Source: CAD feature listing. Evaluate the final solid. Frame: model axes, mm. A direction names the side the tool comes from. Coordinates: 2 decimals unless noted, no trailing zeros. Loops run counter-clockwise (first coordinate to the right, second up) from the corner with the lowest first, then second, coordinate; pieces in that order, holes last.
from build123d import *

# Parameters (mm, degrees)
SKETCH1_W               = 3.175
SKETCH1_H               = 76.2
BOSS_EXTRUDE1_DEPTH     = 12.7
BOSS_EXTRUDE1_2_DEPTH   = 12.7
SKETCH1_3_W             = 12.7
SKETCH1_3_H             = 76.2
SKETCH1_3_W_2           = 3.175
BOSS_EXTRUDE2_DEPTH     = 3.175
FILLET1_R               = 6.35
SKETCH2_W               = 3.175
SKETCH2_H               = 76.2
BOSS_EXTRUDE3_DEPTH     = 9.525
CUT_EXTRUDE1_DEPTH      = 47.878313216
CUT_EXTRUDE1_DEPTH_BACK = 47.878313216
SKETCH3_R               = 2.032
SKETCH4_R               = 1.905
CUT_EXTRUDE2_DEPTH      = 3.175


with BuildPart() as part:
    # Sketch1 → Boss-Extrude1 (new body)
    with BuildSketch(Plane.XY):
        with Locations((-7.9375, 0)):
            Rectangle(SKETCH1_W, SKETCH1_H)
    extrude(amount=BOSS_EXTRUDE1_DEPTH)



with BuildPart() as body_2:
    # Sketch1 → Boss-Extrude1 2 (new body)
    with BuildSketch(Plane.XY):
        with Locations((7.9375, 0)):
            Rectangle(SKETCH1_W, SKETCH1_H)
    extrude(amount=BOSS_EXTRUDE1_2_DEPTH)


with BuildPart() as part_1:
    add(part.part)

    add(body_2.part)  # Boss-Extrude2 merges body 2
    # Sketch1<3> → Boss-Extrude2 (add)
    with BuildSketch(Plane.XY):
        Rectangle(SKETCH1_3_W, SKETCH1_3_H)
        with Locations((7.9375, 0)):
            Rectangle(SKETCH1_3_W_2, SKETCH1_3_H)
        with Locations((-7.9375, 0)):
            Rectangle(SKETCH1_3_W_2, SKETCH1_3_H)
    extrude(amount=-BOSS_EXTRUDE2_DEPTH)

    # Fillet1
    fillet1_edges = [part_1.edges().sort_by_distance(p)[0] for p in [
        (6.35, 0, 0),
        (-6.35, 0, 0),
    ]]
    fillet(fillet1_edges, radius=FILLET1_R - 0.0001)  # a hair under: the kernel refuses the full size

    # Sketch2 → Boss-Extrude3 (add)
    with BuildSketch(Plane.XY.offset(12.7)):
        with Locations((-7.9375, 0)):
            Rectangle(SKETCH2_W, SKETCH2_H)
    extrude(amount=BOSS_EXTRUDE3_DEPTH)

    # Sketch3 → Cut-Extrude1 (cut, two sides: drawn at the far end of the back side and taken through both)
    with BuildSketch(Plane(origin=(-6.35, 0, 0), x_dir=(0, 0, -1), z_dir=(1, 0, 0)).offset(-CUT_EXTRUDE1_DEPTH_BACK)):
        with BuildLine():
            Line((-12.7, 38.1), (-22.225, 38.1))
            Line((-22.225, 38.1), (-22.225, -6.1e-08))
            ThreePointArc((-22.225, -6.1e-08), (-21.749068291, 2.973211742), (-20.368834491, 5.649301068))
            Line((-20.368834491, 5.649301068), (-15.174887346, 12.7))
            ThreePointArc((-15.174887346, 12.7), (-13.334575625, 16.268119062), (-12.7, 20.232401424))
            Line((-12.7, 20.232401424), (-12.7, 38.1))
        make_face()
        with BuildLine():
            ThreePointArc((-20.368834491, -5.649301068), (-21.749068272, -2.973211801), (-22.225, -6.1e-08))
            Line((-22.225, -6.1e-08), (-22.225, -38.1))
            Line((-22.225, -38.1), (-12.7, -38.1))
            Line((-12.7, -38.1), (-12.7, -20.232401424))
            ThreePointArc((-12.7, -20.232401424), (-13.334575625, -16.268119062), (-15.174887346, -12.7))
            Line((-15.174887346, -12.7), (-20.368834491, -5.649301068))
        make_face()
        with Locations((-17.4625, 0)):
            Circle(SKETCH3_R)
    extrude(amount=CUT_EXTRUDE1_DEPTH + CUT_EXTRUDE1_DEPTH_BACK, mode=Mode.SUBTRACT)

    # Sketch4 → Cut-Extrude2 (cut)
    with BuildSketch(Plane.ZY.offset(9.525)):
        with Locations(Location((8.255, 33.655, 0), (0, 0, 270))):
            Circle(SKETCH4_R)
    extrude(amount=-CUT_EXTRUDE2_DEPTH, mode=Mode.SUBTRACT)


solid = part_1.part
Q1. Section D-D, the plane x = -4. Return the cut outline in (y, z) (3 decimals).
Q2. Draft query along Y for faces 1 (the cylindrical face through (-7.96, -16.322, 13.317)), 2 (the flat face through (-9.525, -1, 7)), 3 (the cylindrical face through (-7.96, 35.06, 9.54)). Return one class per face: +Y half, -Y half, draft (parallel to the pull), parting line (faces both ways), or undercut.
Q3. Section C-C, the plane x = -8.25. Count the separate pieces of the cut face and the enclosed holes in it, plus the area to 3 significant figures.
Q4. Access query for faces 4 (the flat face through (-6.35, -1, 11)), 5 (the flat face through (-8, 29, 12.7)), 6 (the flat face through (8, 1, 12.7)). Directions: +Z, -Z, +X, -X, +Y, -Y. A direction counts if a zero-diameter tool reaches every point of the face in a straight line with its end or side. Return the directions, or none.
Q5. Section A-A, the plane z = 11.25. Return the cut outline in (x, y) (3 decimals).
Q6. Line query: line 1 along X through (y, z) = (28, 11) (3 decimals); line 2 along X through (y, z) = (-10.5, 5.25) (3 decimals); line 3 along Z through (x, y) = (-0.25, 9.5) (3 decimals). Output: solid intervals per line, ascending.
Q7. Contact query for flat-ended pins moving along their axis: pin 1 Ø1.6 at (x, y) = (-8.5, 30) entering from +Z; pin 2 Ø5 at (x, z) = (4.5, 14.5) entering from +Y; pin 3 Ø8 at (y, z) = (2, 17) entering from +X. Output: stop coordinate, or through.
Derived:
1. outline: (-38.1, -3.175) - (38.1, -3.175) - (38.1, 1.418) - (-38.1, 1.418) - close
2. face 1: -Y half
2. face 2: draft
2. face 3: undercut
3. separate pieces: 1
3. enclosed holes: 2
3. area: 1,370 mm2
4. face 4: +Z, +Y, -Y
4. face 5: +Z, +X, -X, +Y
4. face 6: +Z, +X, +Y, -Y
5. outline: (-9.525, -38.1) - (-6.35, -38.1) - (-6.35, 38.1) - (-9.525, 38.1) - close; (6.35, -38.1) - (9.525, -38.1) - (9.525, 38.1) - (6.35, 38.1) - close
6. line 1: x = -9.525 to -6.35, 6.35 to 9.525
6. line 2: x = -9.525 to -6.254, 6.254 to 9.525
6. line 3: z = -3.175 to 0.005
7. pin 1: stops at z = 12.7
7. pin 2: passes through
7. pin 3: stops at x = -6.35
